```python
from build123d import *

# Parameters (mm, degrees)
SZKIC3_W                    = 70
SZKIC3_H                    = 370
DODANIE_WYCI_GNI_CIE1_DEPTH = 1.5
WYTNIJ_WYCI_GNI_CIE1_REACH  = 5


with BuildPart() as part:
    # Szkic3 → Dodanie-wyciągnięcie1 (new body, symmetric)
    with BuildSketch(Plane(origin=(0, 0, 113), x_dir=(-1, 0, 0), z_dir=(0, 0, -1))):
        with Locations((95, 0)):
            Rectangle(SZKIC3_W, SZKIC3_H)
    extrude(amount=DODANIE_WYCI_GNI_CIE1_DEPTH, both=True)

    # Szkic4 → Wytnij-wyciągnięcie1 (cut, up to next)
    with BuildSketch(Plane.XY.offset(114.5), mode=Mode.PRIVATE) as wytnij_wyci_gni_cie1_sk1:
        with BuildLine():
            Line((-85.5, -95), (-104.5, -95))
            ThreePointArc((-104.5, -95), (-110.156854249, -92.656854249), (-112.5, -87))
            Line((-112.5, -87), (-112.5, 87))
            ThreePointArc((-112.5, 87), (-110.156854249, 92.656854249), (-104.5, 95))
            Line((-104.5, 95), (-85.5, 95))
            ThreePointArc((-85.5, 95), (-79.843145751, 92.656854249), (-77.5, 87))
            Line((-77.5, 87), (-77.5, -87))
            ThreePointArc((-77.5, -87), (-79.843145751, -92.656854249), (-85.5, -95))
        make_face()
    wytnij_wyci_gni_cie1_tool1 = extrude(wytnij_wyci_gni_cie1_sk1.sketch, amount=-WYTNIJ_WYCI_GNI_CIE1_REACH, mode=Mode.PRIVATE) & part.part
    add(wytnij_wyci_gni_cie1_tool1.solids().sort_by_distance((-95, 0, 114.5))[0], mode=Mode.SUBTRACT)


solid = part.part
```
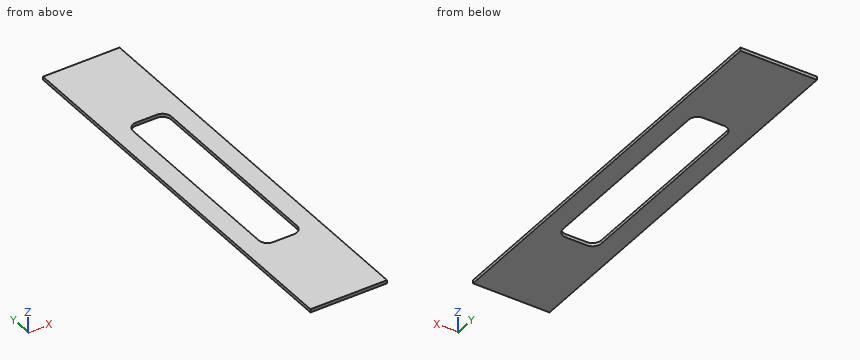
CAD build for the part. Positions are in the model's coordinates, mm. Round coordinates to 2 decimals unless told otherwise and drop trailing zeros. Loops run counter-clockwise (first coordinate to the right, second up) from the corner with the lowest first, then second, coordinate; pieces in that order, holes last. Notation, with made-up numbers: M 7.25,48.25 L 12.25,48.25 A5 ccw 12.25,56.25 Z; hole C 52,-3 d11. An arc over 180 degrees is marked long. Use a Markdown table: item, result. Add a question column.
(1) Cut at B-B (x = -92). Give the cut face in (y, z).
(2) Drill centre lines: line 1 (X direction, y = 79, z = 113.8); line 2 (Y direction, x = -85, z = 114.05); line 3 (Y direction, x = -80.5, z = 112.6) (3 decimals). Where is each one in solid material? Low to high.
(3) Flat gauge pin, fed straight in: pin 1 (12 mm diameter, centred on x = -79, y = 18, fed in from -Z). Where does the tip first touch, or does it go through?
(4) Cut at A-A (z = 113.15). Give the cut face in (x, y), and give its area (3 significant figures).
(5) Cut at C-C (y = 16.5). Give the cut face in (x, z), and give its area (3 significant figures).
Geometry says:
| question | item | result |
|---|---|---|
| 1 | outline | M -185,111.5 L -95,111.5 L -95,114.5 L -185,114.5 Z; M 95,111.5 L 185,111.5 L 185,114.5 L 95,114.5 Z |
| 2 | line 1 | x = -130 to -112.5, -77.5 to -60 |
| 2 | line 2 | y = -185 to -94.98, 94.98 to 185 |
| 2 | line 3 | y = -185 to -93.245, 93.245 to 185 |
| 3 | pin 1 | stops at z = 111.5 |
| 4 | outline | M -130,-185 L -60,-185 L -60,185 L -130,185 Z; hole M -112.5,-87 A8 ccw -104.5,-95 L -85.5,-95 A8 ccw -77.5,-87 L -77.5,87 A8 ccw -85.5,95 L -104.5,95 A8 ccw -112.5,87 Z |
| 4 | area | 19,300 mm² |
| 5 | outline | M -130,111.5 L -112.5,111.5 L -112.5,114.5 L -130,114.5 Z; M -77.5,111.5 L -60,111.5 L -60,114.5 L -77.5,114.5 Z |
| 5 | area | 105 mm² |
